```python
from build123d import *

# Parameters (mm, degrees)
F0_W     = 7.426
F0_H     = 12.45523
F1_DEPTH = 0.75
F3_DEPTH = 7.427


with BuildPart() as f1:
    # F0 (on Right) → F1 (new body)
    with BuildSketch(Plane.YZ):
        with Locations((4.126913, 6.227615)):
            Rectangle(F0_W, F0_H)
    extrude(amount=F1_DEPTH)

    # F2 (on face) → F3 (cut, through all)
    with BuildSketch(Plane.XZ.offset(-0.413913)):
        with BuildLine():
            ThreePointArc((0.57, 0), (0.168979, 1.042876), (0, 2.147347))
            Line((0, 2.147347), (0, 0))
            Line((0, 0), (0.57, 0))
        make_face()
    extrude(amount=-F3_DEPTH, mode=Mode.SUBTRACT)


solid = f1.part
```
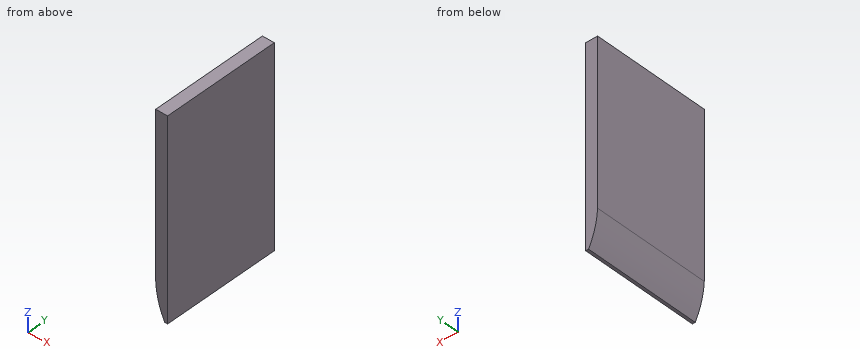
The model under review builds one solid part; all positions refer to its coordinate system, in mm. Round coordinates to 2 decimals unless told otherwise and drop trailing zeros. Loops run counter-clockwise (first coordinate to the right, second up) from the corner with the lowest first, then second, coordinate; pieces in that order, holes last.
1) Consider section C-C on x = 0.45. State the section outline as (y, z) points.
Values follow:
outline: (0.41, 0.25) - (7.84, 0.25) - (7.84, 12.46) - (0.41, 12.46) - close
2) Consider section B-B on z = 1.5. State the section outline as (x, y) points.
Values follow:
outline: (0.07, 0.41) - (0.75, 0.41) - (0.75, 7.84) - (0.07, 7.84) - close
3) Wall thickness on line 1 along X through (y, z) = (6, 1); line 2 along Z through (x, y) = (0.5, 7.25); line 3 along Z through (x, y) = (0.45, 3.5): over which ranges is each line inside the solid? List them lowest first.
Values follow:
line 1: x = 0.18 to 0.75
line 2: z = 0.14 to 12.46
line 3: z = 0.25 to 12.46
4) Consider section A-A on y = 1. State the section outline as (x, z) points.
Values follow:
outline: (0, 2.15) arc R5.2 ccw to (0.57, 0) - (0.75, 0) - (0.75, 12.46) - (0, 12.46) - close
